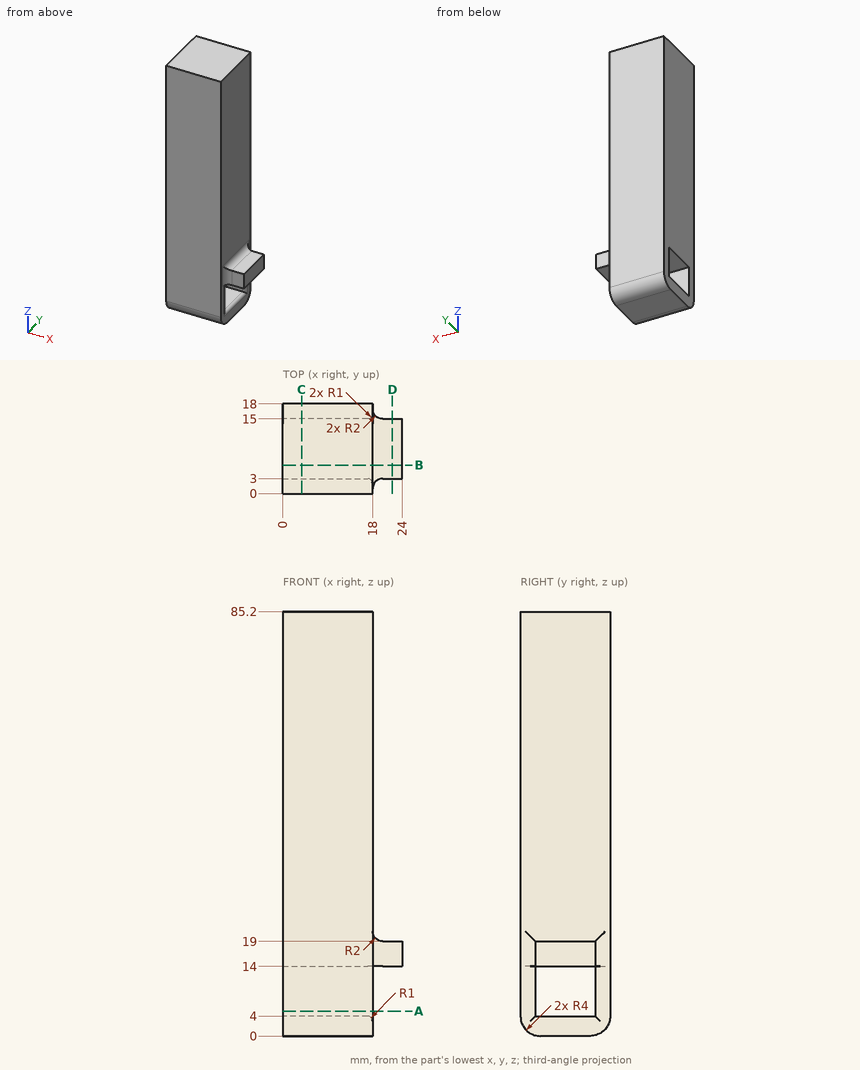
Input: dimensioned drawing with shaded views. Units: mm. Origin: part minimum x, y, z. Give positions to 0.01 mm unless a question says otherwise; leave off trailing zeros. Write each loop counter-clockwise with the first axis right and the second up, starting at its lowest first coordinate (ties: lowest second). Pieces come first, ordered by that corner, then holes. Notation, with made-up numbers: M 49.25,22.25 L 83.25,22.25 A12 ccw 83.25,34.25 Z; hole C 70.25,27 d8. An arc over 180 degrees is marked long. Return JSON: item names as keys, results as strings. Group by question number.
1) Material intervals for line 1 along Z through (x, y) = (13, 4.5); line 2 along Y through (x, z) = (16, 8); line 3 along X through (y, z) = (16, 27), sorted ascending. Write a range as [from, to].
2) Cut plane B-B, the plane y = 5.75. Output: boundary loops of the cut face in (x, z).
3) Cut plane C-C, the plane x = 3.75. Output: boundary loops of the cut face in (y, z), plus the area to 3 significant figures.
4) Pin query (flat end, axial travel): P1, Ø3, axis at x = 22, z = 16, coming from the +Y side; P2, Ø1.2, axis at x = 22, y = 11, coming from the +Z side; P3, Ø1.2, axis at x = 21.5, z = 15.5, coming from the -Y side. Return the tip coordinate at first contact, or that it passes through.
5) Cut plane D-D, the plane x = 22. Output: boundary loops of the cut face in (y, z).
6) Cut plane A-A, the plane z = 5. Output: boundary loops of the cut face in (x, y), plus the area to 3 significant figures.
Recorded:
{
 "1": {"line 1": "z = [0, 4], [14, 85.2]", "line 2": "y = [0, 3], [15, 18]", "line 3": "x = [0, 18]"},
 "2": {"outline": "M 0,0 L 18,0 L 18,3 A1 ccw 17,4 L 0,4 Z; M 0,14 L 24,14 L 24,19 L 20,19 A2 cw 18,21 L 18,85.2 L 0,85.2 Z"},
 "3": {"outline": "M 0,4 A4 ccw 4,0 L 14,0 A4 ccw 18,4 L 18,85.2 L 0,85.2 Z; hole M 3,4 L 15,4 L 15,14 L 3,14 Z", "area": "1,410 mm²"},
 "4": {"P1": "stops at y = 15", "P2": "stops at z = 19", "P3": "stops at y = 3"},
 "5": {"outline": "M 3,14 L 15,14 L 15,19 L 3,19 Z"},
 "6": {"outline": "M 0,0 L 18,0 L 18,2 A1 ccw 17,3 L 0,3 Z; M 0,15 L 17,15 A1 ccw 18,16 L 18,18 L 0,18 Z", "area": "108 mm²"}
}
